The drawing under review shows one solid part. Ordinate dimensions are in mm from its lowest x, y, z. A direction names the side the tool comes from. Coordinates: 2 decimals unless noted, no trailing zeros. Loops run counter-clockwise (first coordinate to the right, second up) from the corner with the lowest first, then second, coordinate; pieces in that order, holes last. Notation, with made-up numbers: (21, -22) - (53, -22) arc R20 ccw to (53, -4) - close; hole circle Ø1 at (-31.75, -28.75). An arc over 180 degrees is marked (long way). Answer as a JSON object with one key per item and string values. Group by question number.
Item 1: We need section C-C (z = 41.5). Give the boundary of the cut face in (x, y), then the cut area to 3 significant figures.
Item 2: We need section D-D (y = 27). Give the boundary of the cut face in (x, z), then the cut area to 3 significant figures.
Item 3: Mouldability with a two-part tool opening along X and no side actions: class the marked faces 1, 2, 3 and 4 as released by +X, released by -X, zero draft, split by the parting line, or undercut.
Item 4: We need section A-A (x = 52). Give the boundary of the cut face in (y, z).
Item 5: Tool access review of the marked faces 5, 6 and 7: name each direction out of +Z, -Z, +X, -X, +Y, -Y from which nothing blocks a thin tool from reaching the whole face with its end or side.
Item 6: Clearance check with flat-ended pins moving along their axes: pin 1 (2 mm diameter, centred on y = 77.5, z = 51, fed in from +X); pin 2 (12 mm diameter, centred on x = 46.5, y = 49.5, fed in from +Z); pin 3 (10 mm diameter, centred on x = 72.5, z = 48.5, fed in from +Y); pin 4 (17.5 mm diameter, centred on x = 52, y = 52, fed in from +Z). State where each tip first meets the part, or that it passes through.
Item 7: To check wall thickness, follow line 1 (Y direction, x = 52, z = 22); line 2 (Z direction, x = 91, y = 18); line 3 (Z direction, x = 47.5, y = 67.5). State the ranges of each line that lie inside material, in increasing order.
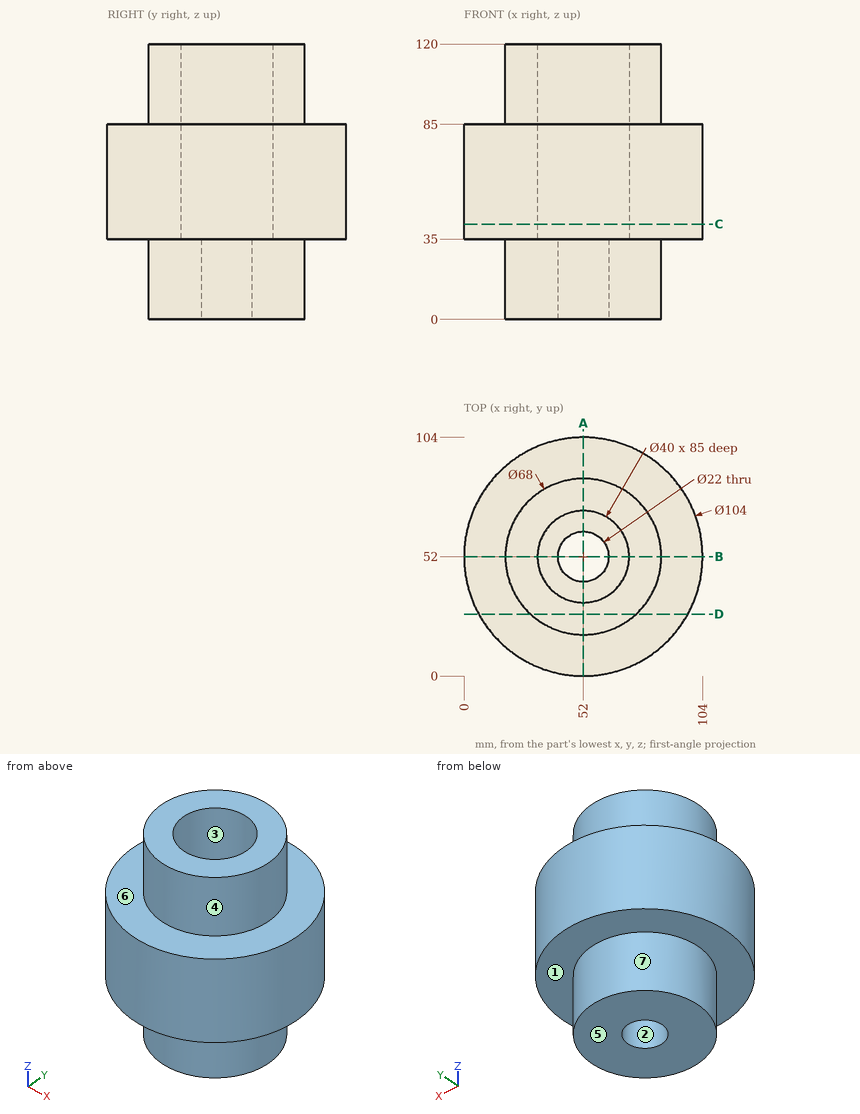
Check sheet entries:
{
 "1": {"outline": "circle Ø104 at (52, 52); hole circle Ø40 at (52, 52)", "area": "7,240 mm2"},
 "2": {"outline": "(6.4, 35) - (28.96, 35) - (28.96, 0) - (75.04, 0) - (75.04, 35) - (97.6, 35) - (97.6, 85) - (75.04, 85) - (75.04, 120) - (28.96, 120) - (28.96, 85) - (6.4, 85) - close", "area": "7,790 mm2"},
 "3": {"face 1": "zero draft", "face 2": "undercut", "face 3": "undercut", "face 4": "split by the parting line"},
 "4": {"outline": "(0, 35) - (18, 35) - (18, 0) - (41, 0) - (41, 35) - (32, 35) - (32, 120) - (18, 120) - (18, 85) - (0, 85) - close; (63, 0) - (86, 0) - (86, 35) - (104, 35) - (104, 85) - (86, 85) - (86, 120) - (72, 120) - (72, 35) - (63, 35) - close"},
 "5": {"face 5": "-Z, +X, -X, +Y, -Y", "face 6": "+Z", "face 7": "-Z"},
 "6": {"pin 1": "stops at x = 97.87", "pin 2": "stops at z = 35", "pin 3": "stops at y = 101.64", "pin 4": "passes through"},
 "7": {"line 1": "y = 18 to 41, 63 to 86", "line 2": "z = 35 to 85", "line 3": "z = 0 to 35"}
}
